from build123d import *

# Parameters (mm, degrees)
SKETCH1_W           = 142.367
SKETCH1_H           = 68.58
BOSS_EXTRUDE1_DEPTH = 6
SKETCH2_W           = 5.588
SKETCH2_H           = 4.1275
BOSS_EXTRUDE2_DEPTH = 6
BOSS_EXTRUDE3_DEPTH = 6
CUT_EXTRUDE1_DEPTH  = 160.827015204
BOSS_EXTRUDE4_DEPTH = 6
SKETCH6_R           = 1.778
SKETCH6_R_2         = 1.5875
CUT_EXTRUDE2_DEPTH  = 161.845851191


with BuildPart() as part:
    # Sketch1 → Boss-Extrude1 (new body)
    with BuildSketch(Plane.XY):
        with Locations((71.1835, 34.29)):
            Rectangle(SKETCH1_W, SKETCH1_H)
    extrude(amount=BOSS_EXTRUDE1_DEPTH)

    # Sketch2 → Boss-Extrude2 (add)
    with BuildSketch(Plane.XY.offset(6)):
        with Locations((-2.794, 66.51625)):
            Rectangle(SKETCH2_W, SKETCH2_H)
        with Locations((-2.794, 2.06375)):
            Rectangle(SKETCH2_W, SKETCH2_H)
    extrude(amount=-BOSS_EXTRUDE2_DEPTH)

    # Sketch3 → Boss-Extrude3 (add)
    with BuildSketch(Plane.XY.offset(6)):
        Polygon((0, 68.58), (0, 72.39), (2.54, 72.39), (9.525, 68.58), align=None)
        Polygon((0, 0), (0, -3.81), (2.54, -3.81), (9.525, 0), align=None)
    extrude(amount=-BOSS_EXTRUDE3_DEPTH)

    # Sketch4 → Cut-Extrude1 (cut, through all)
    with BuildSketch(Plane.XY.offset(6)):
        Polygon((142.367, 44.958), (136.017, 44.958), (136.017, 47.14875), (132.842, 47.14875), (132.842, 39.21125), (136.017, 39.21125), (136.017, 41.402), (142.367, 41.402), align=None)
        Polygon((142.367, 14.478), (136.017, 14.478), (136.017, 16.66875), (132.842, 16.66875), (132.842, 8.73125), (136.017, 8.73125), (136.017, 10.922), (142.367, 10.922), align=None)
        Polygon((93.9038, 62.23), (91.71305, 62.23), (91.71305, 59.055), (99.65055, 59.055), (99.65055, 62.23), (97.4598, 62.23), (97.4598, 68.58), (93.9038, 68.58), align=None)
        Polygon((123.33224, 68.58), (119.77624, 68.58), (119.77624, 62.23), (117.58549, 62.23), (117.58549, 59.055), (125.52299, 59.055), (125.52299, 62.23), (123.33224, 62.23), align=None)
    extrude(amount=-CUT_EXTRUDE1_DEPTH, mode=Mode.SUBTRACT)

    # Sketch5 → Boss-Extrude4 (add)
    with BuildSketch(Plane.XY.offset(6)):
        Polygon((10.287, 0), (3.937, -6.0325), (-5.588, -6.0325), (-5.588, 0), align=None)
        Polygon((-5.588, 68.58), (10.287, 68.58), (3.937, 74.6125), (-5.588, 74.6125), align=None)
    extrude(amount=-BOSS_EXTRUDE4_DEPTH)

    # Sketch6 → Cut-Extrude2 (cut, through all)
    with BuildSketch(Plane.XY.offset(6)):
        with Locations((-2.413, 68.5165)):
            Circle(SKETCH6_R)
        with Locations((-2.413, 0.0635)):
            Circle(SKETCH6_R)
        with Locations((64.77, 3.81)):
            Circle(SKETCH6_R_2)
        with Locations((72.39, 3.81)):
            Circle(SKETCH6_R_2)
        with Locations((41.275, 3.81)):
            Circle(SKETCH6_R_2)
        with Locations((48.895, 3.81)):
            Circle(SKETCH6_R_2)
        with Locations((41.275, 10.16)):
            Circle(SKETCH6_R_2)
        with Locations((48.895, 10.16)):
            Circle(SKETCH6_R_2)
    extrude(amount=-CUT_EXTRUDE2_DEPTH, mode=Mode.SUBTRACT)


solid = part.part
For this review, take the finished solid that the model builds, in its own axes (mm). A direction names the side the tool comes from. Round coordinates to 2 decimals unless told otherwise and drop trailing zeros. Order: outer loops, then holes, each group sorted by start corner. A loop starts at its lowest first (then second) coordinate and runs counter-clockwise, first axis right, second up. Notation, with made-up numbers: (20, 19) -> (50, 19) arc R18 cw to (50, 43) -> close; hole circle Ø4 at (-37, -33). An arc over 180 degrees is marked (long way). Put each result on its own line as item: value.
Q1. Add section C-C on x = 127.5. Write out the cut boundary in (y, z), plus the area to 3 significant figures.
Check result:
outline: (0, 0) -> (68.58, 0) -> (68.58, 6) -> (0, 6) -> close
area: 411 mm2
Q2. Mouldability with a two-part tool opening along Y and no side actions: class faces 1 (the flat face through (75, 0, 3)), 2 (the flat face through (142.367, 28, 3)), 3 (the cylindrical face through (42.79, 4.29, 3.04)), 4 (the flat face through (-3, 64.452, 3)) as pulls with the +Y half, pulls with the -Y half, needs draft (parallel to the pull), parting line crosses it, or undercut.
Check result:
face 1: pulls with the -Y half
face 2: needs draft
face 3: undercut
face 4: undercut
Q3. For probe 1 along X at (y, z) = (61, 1.25); probe 2 along Y at (x, z) = (125, 5.5) (3 decimals); probe 3 along Y at (x, z) = (72.39, 3.15), list the stretches that pass through material, from the lowest coordinate up. Write a range as [from, to].
Check result:
probe 1: [0, 91.71], [99.65, 117.59], [125.52, 142.37]
probe 2: [0, 59.055], [62.23, 68.58]
probe 3: [0, 2.22], [5.4, 68.58]
Q4. Insertion check: pin 1 Ø2.5 at (x, z) = (93.5, 3.5) entering from -Y; pin 2 Ø3 at (x, z) = (97.5, 3.5) entering from +Y. Each pin has a flat end and moves straight along its axis. Give the tip position at first contact, or say it passes through.
Check result:
pin 1: y = 0
pin 2: y = 68.58
Q5. Machinability: for faces 5 (the flat face through (134, 8.731, 3)), 6 (the flat face through (93.904, 65, 3)), 7 (the flat face through (133, 68.58, 3)), which of the approach directions +Z, -Z, +X, -X, +Y, -Y give a long, thin tool a straight path to every point of the face, cutting with its end or side? Answer none if there is none.
Check result:
face 5: +Z, -Z
face 6: +Z, -Z, +Y
face 7: +Z, -Z, +X, +Y
Q6. Add section B-B on y = 29. Write out the cut boundary in (x, z), plus the area to 3 significant figures.
Check result:
outline: (0, 0) -> (142.37, 0) -> (142.37, 6) -> (0, 6) -> close
area: 854 mm2
Q7. Add section A-A on x = 72.39. Write out the cut boundary in (y, z), plus the area to 3 significant figures.
Check result:
outline: (0, 0) -> (2.22, 0) -> (2.22, 6) -> (0, 6) -> close; (5.4, 0) -> (68.58, 0) -> (68.58, 6) -> (5.4, 6) -> close
area: 392 mm2
Q8. Add section D-D on z = 1.25. State how many separate pieces and enclosed holes the cut face has, plus the area to 3 significant figures.
Check result:
separate pieces: 1
enclosed holes: 8
area: 9,700 mm2
